from build123d import *

# Parameters (mm, degrees)
F0_W     = 147.32
F0_H     = 147.32
F0_W_2   = 121.92
F0_H_2   = 121.92
F1_DEPTH = 63.5
F2_W     = 132.08
F2_H     = 132.08
F3_DEPTH = 101.6
F4_SIZE  = 2.54
F5_SIZE  = 5.08


with BuildPart() as f1:
    # F0 (on Top) → F1 (new body, symmetric)
    with BuildSketch(Plane.XY):
        Rectangle(F0_W, F0_H)
        Rectangle(F0_W_2, F0_H_2, mode=Mode.SUBTRACT)
        Rectangle(F0_W_2, F0_H_2)
    extrude(amount=F1_DEPTH, both=True)

    # F2 (on face) → F3 (cut)
    with BuildSketch(Plane.XY.offset(63.5)):
        Rectangle(F2_W, F2_H)
    extrude(amount=-F3_DEPTH, mode=Mode.SUBTRACT)

    # F4
    f4_edges = [f1.edges().sort_by_distance(p)[0] for p in [
        (-73.66, -73.66, 0),
        (-73.66, 0, 63.5),
        (-73.66, 73.66, 0),
        (-73.66, 0, -63.5),
        (0, -73.66, 63.5),
        (73.66, -73.66, 0),
        (0, -73.66, -63.5),
        (66.04, 0, 63.5),
        (0, -66.04, 63.5),
        (73.66, 0, 63.5),
        (73.66, 0, -63.5),
        (73.66, 73.66, 0),
        (0, 73.66, 63.5),
        (0, 73.66, -63.5),
        (-66.04, 0, 63.5),
        (0, 66.04, 63.5),
        (0, -66.04, -38.1),
    ]]
    chamfer(f4_edges, length=F4_SIZE)

    # F5
    f5_edges = [f1.edges().sort_by_distance(p)[0] for p in [
        (66.04, 1.27, -38.1),
        (0, 66.04, -38.1),
        (-66.04, 1.27, -38.1),
    ]]
    chamfer(f5_edges, length=F5_SIZE)


solid = f1.part
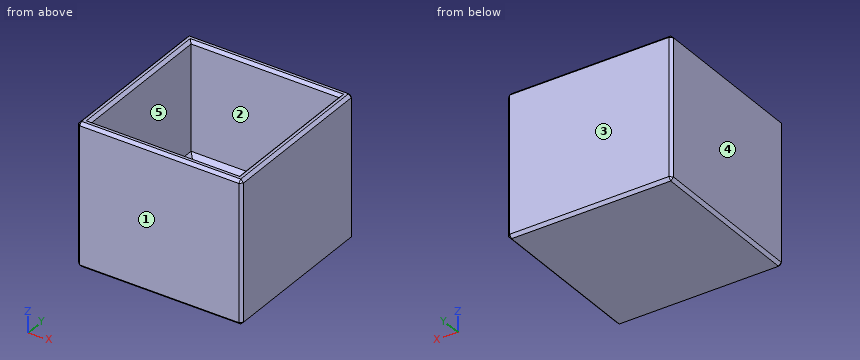
The listing builds one solid part. Answer for the finished solid, in the listing's coordinates (mm). Face numbers are marked on the shaded views. A direction names the side the tool comes from. Coordinates: 2 decimals unless noted, no trailing zeros. Order: outer loops, then holes, each group sorted by start corner. A loop starts at its lowest first (then second) coordinate and runs counter-clockwise, first axis right, second up.
Q1. Given P1, Ø12, axis at x = -32.5, y = 47, coming from the +Z side, flat-ended and moving along its own axis, determine where the tip first touches the part or whether it passes through.
Q2. A cutting plane is placed at A-A, the plane z = 46. Write down the section's boundary in (x, y), and give its area (3 significant figures).
Q3. Consider line 1 (Y direction, x = 40.5, z = -2); line 2 (Z direction, x = 50, y = -31.5). Determine where each line is inside the solid, lowest interval first.
Q4. Which of the six approach directions +Z, -Z, +X, -X, +Y, -Y give full straight-line access (tool end or side, diameter ignored) to the marked faces 1 and 2?
Q5. A cutting plane is placed at B-B, the plane x = 4. Write down the section's boundary in (y, z), and give its area (3 significant figures).
Q6. A cutting plane is placed at C-C, the plane y = 8. Write down the section's boundary in (x, z), and give its area (3 significant figures).
Q7. For a pull along X with two mould halves and no side action, classify the marked faces 3, 4 and 5 as pulls with the +X half, pulls with the -X half, needs draft (parallel to the pull), parting line crosses it, or undercut.
Answers follow:
1. P1: stops at z = -38.1
2. outline: (-73.66, -71.12) - (-71.12, -73.66) - (71.12, -73.66) - (73.66, -71.12) - (73.66, 71.12) - (71.12, 73.66) - (-71.12, 73.66) - (-73.66, 71.12) - close; hole (-66.04, -66.04) - (66.04, -66.04) - (66.04, 66.04) - (-66.04, 66.04) - close
2. area: 4,250 mm2
3. line 1: y = -73.66 to -66.04, 66.04 to 73.66
3. line 2: z = -63.5 to -38.1
4. face 1: +Z, -Z, +X, -X, -Y
4. face 2: +Z
5. outline: (-73.66, -60.96) - (-71.12, -63.5) - (71.12, -63.5) - (73.66, -60.96) - (73.66, 60.96) - (71.12, 63.5) - (68.58, 63.5) - (66.04, 60.96) - (66.04, -33.02) - (60.96, -38.1) - (-63.5, -38.1) - (-66.04, -35.56) - (-66.04, 60.96) - (-68.58, 63.5) - (-71.12, 63.5) - (-73.66, 60.96) - close
5. area: 5,290 mm2
6. outline: (-73.66, -60.96) - (-71.12, -63.5) - (71.12, -63.5) - (73.66, -60.96) - (73.66, 60.96) - (71.12, 63.5) - (68.58, 63.5) - (66.04, 60.96) - (66.04, -33.02) - (60.96, -38.1) - (-60.96, -38.1) - (-66.04, -33.02) - (-66.04, 60.96) - (-68.58, 63.5) - (-71.12, 63.5) - (-73.66, 60.96) - close
6. area: 5,300 mm2
7. face 3: needs draft
7. face 4: pulls with the -X half
7. face 5: undercut
